Source: three-view drawing plus pictorial views. Frame: mm from the lowest corner of the part. A direction names the side the tool comes from. Give positions to 0.01 mm unless a question says otherwise; leave off trailing zeros. Order: outer loops, then holes, each group sorted by start corner. A loop starts at its lowest first (then second) coordinate and runs counter-clockwise, first axis right, second up.
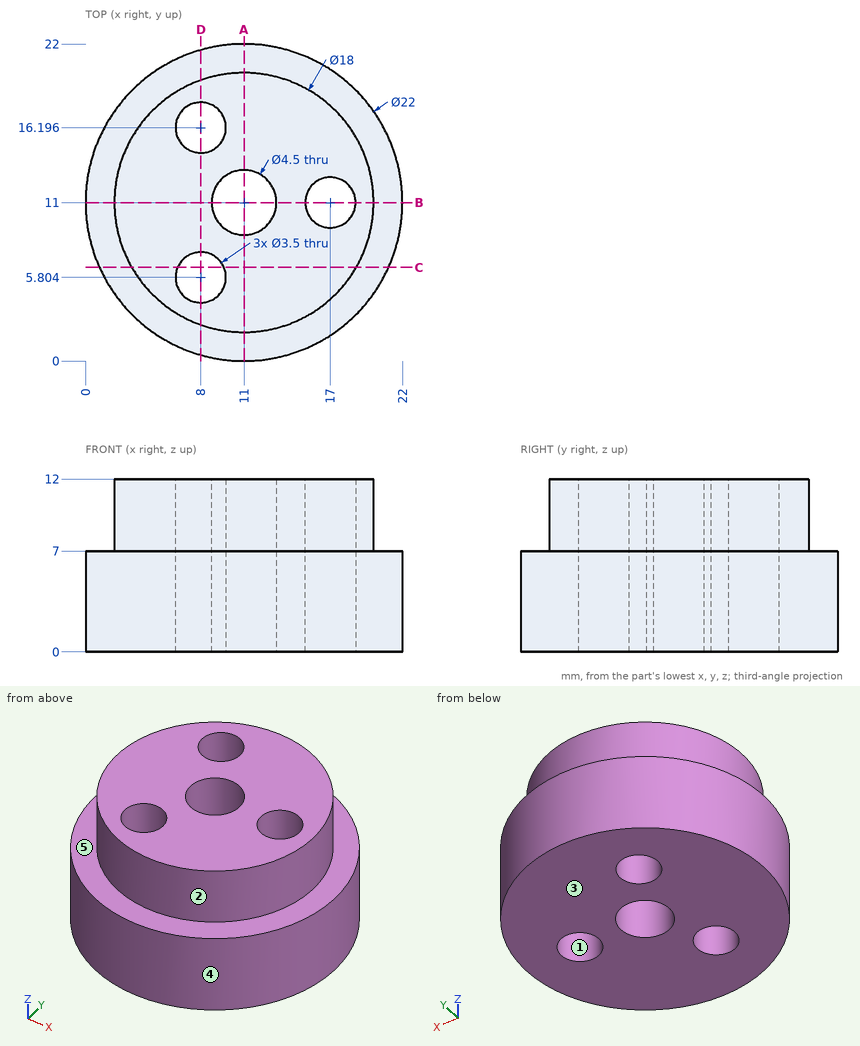
(1) Pin query (flat end, axial travel): pin 1 Ø4.5 at (x, y) = (8, 16.2) entering from +Z; pin 2 Ø1.5 at (y, z) = (3.5, 5.5) entering from +X (1 decimal); pin 3 Ø3 at (x, y) = (17.5, 2) entering from +Z. Return the tip coordinate at first contact, or that it passes through.
(2) Line query: line 1 along Y through (x, z) = (7.5, 3.5); line 2 along Y through (x, z) = (8, 7.75) (1 decimal); line 3 along X through (y, z) = (17.25, 10.75) (1 decimal). Output: solid intervals per line, ascending.
(3) Access query for the marked faces 4 and 5. Directions: +Z, -Z, +X, -X, +Y, -Y. A direction counts if a zero-diameter tool reaches every point of the face in a straight line with its end or side. Return the directions, or none.
(4) Section D-D, the plane x = 8. Return loops of the section in (y, z) (1 decimal).
(5) Section C-C, the plane y = 6.5. Return loops of the section in (x, z).
(6) Section B-B, the plane y = 11. Return loops of the section in (x, z).
(7) Draft query along Y for the marked faces 1, 2 and 3. Return one class per face: +Y half, -Y half, draft (parallel to the pull), parting line (faces both ways), or undercut.
(8) Section A-A, the plane x = 11. Return loops of the section in (y, z).
Checks:
1. pin 1: stops at z = 12
1. pin 2: stops at x = 19.7
1. pin 3: stops at z = 7
2. line 1: y = 0.57 to 4.13, 7.48 to 14.52, 17.87 to 21.43
2. line 2: y = 2.5 to 4.1, 7.6 to 14.4, 17.9 to 19.5
2. line 3: x = 4.5 to 6.6, 9.4 to 17.5
3. face 4: +Z, -Z
3. face 5: +Z
4. outline: (0.4, 0) - (4.1, 0) - (4.1, 12) - (2.5, 12) - (2.5, 7) - (0.4, 7) - close; (7.6, 0) - (14.4, 0) - (14.4, 12) - (7.6, 12) - close; (17.9, 0) - (21.6, 0) - (21.6, 7) - (19.5, 7) - (19.5, 12) - (17.9, 12) - close
5. outline: (0.96, 0) - (6.39, 0) - (6.39, 12) - (3.21, 12) - (3.21, 7) - (0.96, 7) - close; (9.61, 0) - (21.04, 0) - (21.04, 7) - (18.79, 7) - (18.79, 12) - (9.61, 12) - close
6. outline: (0, 0) - (8.75, 0) - (8.75, 12) - (2, 12) - (2, 7) - (0, 7) - close; (13.25, 0) - (15.25, 0) - (15.25, 12) - (13.25, 12) - close; (18.75, 0) - (22, 0) - (22, 7) - (20, 7) - (20, 12) - (18.75, 12) - close
7. face 1: undercut
7. face 2: parting line
7. face 3: draft
8. outline: (0, 0) - (8.75, 0) - (8.75, 12) - (2, 12) - (2, 7) - (0, 7) - close; (13.25, 0) - (22, 0) - (22, 7) - (20, 7) - (20, 12) - (13.25, 12) - close
